Autodesk Inventor part; units mm, degrees
ref_plane "YZ Plane" through (0, 0, 0) normal (1, 0, 0) x (0, 1, 0)
ref_plane "XZ Plane" through (0, 0, 0) normal (0, 1, 0) x (-1, 0, 0)
ref_plane "XY Plane" through (0, 0, 0) normal (0, 0, 1) x (1, 0, 0)
sketch "Sketch1" plane through (0, 0, 0) normal (0, 1, 0) x (-1, 0, 0)
  line L0 (-7.5, 6.6144) -> (7.5, 6.6144) construction
  line L1 (7.5, 6.6144) -> (7.5, -6.6144)
  line L2 (7.5, -6.6144) -> (-7.5, -6.6144) construction
  line L3 (-7.5, -6.6144) -> (-7.5, 6.6144)
  line L4 (-7.5, 6.6144) -> (7.5, -6.6144) construction
  line L5 (7.5, 6.6144) -> (-7.5, -6.6144) construction
  arc A0 (7.5, 6.6144) -> (-7.5, 6.6144) centre (0, 0) ccw
  arc A1 (-7.5, -6.6144) -> (7.5, -6.6144) centre (0, 0) ccw
  line L6 (-12.5, 8.2916) -> (-12.5, -8.2916)
  arc A2 (-12.5, -8.2916) -> (12.5, -8.2916) centre (0, 0) ccw
  line L7 (12.5, -8.2916) -> (12.5, 8.2916)
  arc A3 (12.5, 8.2916) -> (-12.5, 8.2916) centre (0, 0) ccw
  dimension "d1" = 15
  dimension "d2" = 10
  dimension "d3" = 5
extrude "Extrusion1" add sketch "Sketch1" along normal blind 25
sketch "Sketch2" plane through (0, 25, 0) normal (0, 1, 0) x (1, 0, 0)
  arc A0 (12.5, 8.2916) -> (-12.5, 8.2916) centre (0, 0) ccw
  line L0 (-12.5, 8.2916) -> (-12.5, -8.2916)
  arc A1 (-12.5, -8.2916) -> (12.5, -8.2916) centre (0, 0) ccw
  line L1 (12.5, -8.2916) -> (12.5, 8.2916)
  line L2 (7.5, 6.6144) -> (7.5, -6.6144)
  arc A2 (-7.5, -6.6144) -> (7.5, -6.6144) centre (0, 0) ccw
  line L3 (-7.5, -6.6144) -> (-7.5, 6.6144)
  arc A3 (7.5, 6.6144) -> (-7.5, 6.6144) centre (0, 0) ccw
  circle A4 centre (0, 0) radius 6
  dimension "d6" = 12
extrude "Extrusion2" add sketch "Sketch2" along normal blind 5 contours L1 A1 L0 A0 | L2 A2 L3 A3
sketch "Sketch3" plane through (12.5, 0, 8.2916) normal (1, 0, 0) x (0, 0, -1)
  line L0 (18.2916, 18) -> (-1.7084, 18)
  line L1 (-1.7084, 18) -> (-1.7084, 30)
  line L2 (-1.7084, 30) -> (18.2916, 30)
  line L3 (18.2916, 30) -> (18.2916, 18)
  line L4 (0, 30) -> (16.5831, 30)
  point P0 (8.2916, 0)
  point P1 (8.2916, 30)
  dimension "d9" = 12
  dimension "d10" = 20
extrude "Extrusion3" cut sketch "Sketch3" against normal blind 6
sketch "Sketch4" plane through (12.5, 18, 8.2916) normal (0, 1, 0) x (1, 0, 0)
  arc A0 (-1.3197, -1.7084) -> (0, 0) centre (-12.5, 8.2916) ccw
  line L0 (0, 16.5831) -> (0, 0)
  arc A1 (0, 16.5831) -> (-1.3197, 18.2916) centre (-12.5, 8.2916) ccw
  line L1 (-1.3197, 18.2916) -> (-6, 18.2916)
  line L2 (-6, 18.2916) -> (-6, 15.8909)
  arc A2 (-5, 14.9059) -> (-6, 15.8909) centre (-12.5, 8.2916) ccw
  line L3 (-5, 1.6772) -> (-5, 14.9059)
  arc A3 (-6, 0.6922) -> (-5, 1.6772) centre (-12.5, 8.2916) ccw
  line L4 (-6, 0.6922) -> (-6, -1.7084)
  line L5 (-1.3197, -1.7084) -> (-6, -1.7084)
  point P0 (-12.5, 8.2916)
extrude "Extrusion4" cut sketch "Sketch4" against normal through all
sketch "Sketch5" plane through (0, 0, 0) normal (0, -1, 0) x (1, 0, 0)
  line L0 (6.5, -10) -> (6.5, -7.5993)
  arc A0 (-7.5, -6.6144) -> (6.5, -7.5993) centre (0, 0) ccw
  line L1 (-7.5, 6.6144) -> (-7.5, -6.6144)
  arc A1 (6.5, 7.5993) -> (-7.5, 6.6144) centre (0, 0) ccw
  line L2 (6.5, 7.5993) -> (6.5, 10)
  line L3 (6.5, 10) -> (11.1803, 10)
  arc A2 (11.1803, 10) -> (-12.5, 8.2916) centre (0, 0) ccw
  line L4 (-12.5, -8.2916) -> (-12.5, 8.2916)
  arc A3 (-12.5, -8.2916) -> (11.1803, -10) centre (0, 0) ccw
  line L5 (11.1803, -10) -> (6.5, -10)
  line L6 (0, 25) -> (0, -25)
  circle A4 centre (0, 25) radius 5
  circle A5 centre (0, -25) radius 5
  line L7 (4.6617, 26.8079) -> (11.1803, 10)
  line L8 (11.1803, -10) -> (4.6617, -26.8079)
  line L9 (-4.6047, -26.9486) -> (-12.5, -8.2916)
  line L10 (-12.5, 8.2916) -> (-4.6047, 26.9486)
  dimension "d15" = 50
  dimension "d16" = 10
  dimension "d17" = 10
extrude "Extrusion5" add sketch "Sketch5" against normal blind 5 contours L8 A5 L6 A3 | L6 A5 L9 A3 | A5 | L6 A4 L7 A2 | A2 L10 A4 L6 | A4
sketch "Sketch6" plane through (0, 5, 0) normal (0, 1, 0) x (1, 0, 0)
  line L0 (-12.5, -8.2916) -> (-4.6047, -26.9486)
  arc A0 (-4.6047, -26.9486) -> (4.6617, -26.8079) centre (0, -25) ccw
  line L1 (4.6617, -26.8079) -> (11.1803, -10)
  arc A1 (-12.5, -8.2916) -> (11.1803, -10) centre (0, 0) ccw
  arc A2 (11.1803, 10) -> (-12.5, 8.2916) centre (0, 0) ccw
  line L2 (11.1803, 10) -> (4.6617, 26.8079)
  arc A3 (4.6617, 26.8079) -> (-4.6047, 26.9486) centre (0, 25) ccw
  line L3 (-4.6047, 26.9486) -> (-12.5, 8.2916)
hole "Hole1" at (0, 5, 25) at (0, 5, -25) direction (0, -1, 0) diameter 3.4 end through all counterbore diameter 6.5 counterbore depth 3.4
properties part number "motor mount"
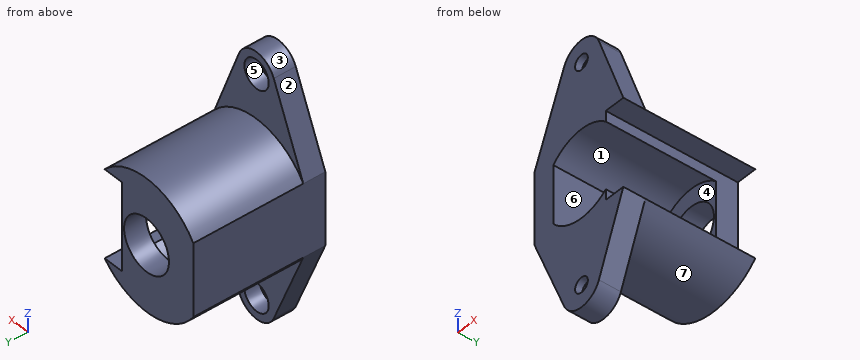
The listing builds one solid part. Answer for the finished solid, in the listing's coordinates (mm). Face numbers are marked on the shaded views. A direction names the side the tool comes from. Coordinates: 2 decimals unless noted, no trailing zeros. Order: outer loops, then holes, each group sorted by start corner. A loop starts at its lowest first (then second) coordinate and runs counter-clockwise, first axis right, second up.
Q1. A cutting plane is placed at B-B, the plane x = 0. State how many separate pieces and enclosed holes the cut face has, and give its area (3 significant figures).
Q2. Which of the six approach directions +Z, -Z, +X, -X, +Y, -Y give full straight-line access (tool end or side, diameter ignored) to the marked faces 4, 5, 6 and 7?
Q3. For a pull along X with two mould halves and no side action, classify the marked faces 1, 2 and 3 as pulls with the +X half, pulls with the -X half, needs draft (parallel to the pull), parting line crosses it, or undercut.
Q4. A cutting plane is placed at A-A, the plane z = 0. Write down the section's boundary in (x, y), and give its area (3 significant figures).
Q5. A cutting plane is placed at C-C, the plane y = 3. Write down the section's boundary in (x, z), and give its area (3 significant figures).
Q6. A cutting plane is placed at D-D, the plane z = -22.5. Write down the section's boundary in (x, y).
Q7. Consider line 1 (Z direction, x = 0, y = 0.7); line 2 (Z direction, x = 0, y = 4.25); line 3 (X direction, y = 28.6, z = 0). Determine where each line is inside the solid, lowest interval first.
Q8. Given P1, Ø1.4, axis at x = 10, y = 13.5, coming from the -Z side; P2, Ø7, axis at x = 2.5, z = 3, coming from the -Y side; P3, Ø7, axis at x = -1, z = -26, coming from the +Y side; P4, Ø5.5, axis at x = 0, z = 25, coming from the -Y side, each flat-ended and moving along its own axis, determine where each tip first touches the part or whether it passes through.
Answers follow:
1. separate pieces: 4
1. enclosed holes: 0
1. area: 435 mm2
2. face 4: -Y
2. face 5: +Y
2. face 6: +X, -Y
2. face 7: -Z, +Y
3. face 1: undercut
3. face 2: pulls with the -X half
3. face 3: parting line crosses it
4. outline: (-12.5, 0) - (-7.5, 0) - (-7.5, 25) - (-6, 25) - (-6, 30) - (-12.5, 30) - close; (6, 25) - (6.5, 25) - (6.5, 30) - (6, 30) - close
4. area: 160 mm2
5. outline: (-12.5, -8.29) - (-4.6, -26.95) arc R5 ccw to (4.66, -26.81) - (11.18, -10) - (6.5, -10) - (6.5, -7.6) arc R10 cw to (-7.5, -6.61) - (-7.5, 6.61) arc R10 cw to (6.5, 7.6) - (6.5, 10) - (11.18, 10) - (4.66, 26.81) arc R5 ccw to (-4.6, 26.95) - (-12.5, 8.29) - close; hole circle Ø6.5 at (0, -25); hole circle Ø6.5 at (0, 25)
5. area: 644 mm2
6. outline: (-6.49, 0) - (6.33, 0) - (6.33, 5) - (2.08, 5) - (2.08, 1.6) - (-2.08, 1.6) - (-2.08, 5) - (-6.49, 5) - close
7. line 1: z = -30 to -26.7, -23.3 to -10, 10 to 23.3, 26.7 to 30
7. line 2: z = -30 to -28.25, -21.75 to -10, 10 to 21.75, 28.25 to 30
7. line 3: x = -12.5 to -6, 6 to 6.5
8. P1: stops at z = -11.77
8. P2: stops at y = 25
8. P3: stops at y = 5
8. P4: stops at y = 0
